Here's how the part is built. I have some questions about the finished solid (model axes, mm). Face numbers are marked on the shaded views. A direction names the side the tool comes from. Round coordinates to 2 decimals unless told otherwise and drop trailing zeros. Loops run counter-clockwise (first coordinate to the right, second up) from the corner with the lowest first, then second, coordinate; pieces in that order, holes last. Notation, with made-up numbers: M 43.5,0.5 L 74.5,0.5 A19 cw 74.5,31.5 Z; hole C 16,66.5 d7. An arc over 180 degrees is marked long. Write each question's results on one line, items separated by ' | '. Start each with the question number.
Autodesk Inventor part; units mm, degrees
ref_plane "YZ Plane" through (0, 0, 0) normal (1, 0, 0) x (0, 1, 0)
ref_plane "XZ Plane" through (0, 0, 0) normal (0, 1, 0) x (-1, 0, 0)
ref_plane "XY Plane" through (0, 0, 0) normal (0, 0, 1) x (1, 0, 0)
sketch "草图1" plane through (0, 0, 0) normal (0, 1, 0) x (-1, 0, 0)
  line L0 (65, 82) -> (-65, 82)
  line L1 (-65, 82) -> (-65, -82)
  line L2 (-65, -82) -> (65, -82)
  line L3 (65, -82) -> (65, 82)
  line L4 (65, 82) -> (-65, -82) construction
  line L5 (-65, 82) -> (65, -82) construction
  point P0 (0, 0)
  dimension "d0" = 130
  dimension "d1" = 164
extrude "拉伸1" add sketch "草图1" along normal blind 15
sketch "草图2" plane through (0, 15, 0) normal (0, 1, 0) x (1, 0, 0)
  line L0 (-40, -82) -> (40, -82)
  line L1 (40, -82) -> (40, 82)
  line L2 (40, 82) -> (-40, 82)
  line L3 (-40, 82) -> (-40, -82)
  line L4 (-40, -82) -> (40, 82) construction
  line L5 (40, -82) -> (-40, 82) construction
  point P0 (0, 0)
  dimension "d4" = 80
  dimension "d5" = 164
extrude "拉伸2" add sketch "草图2" along normal blind 65
sketch "草图3" plane through (0, 0, 0) normal (0, -1, 0) x (1, 0, 0)
  line L0 (34.5, 82) -> (-34.5, 82)
  line L1 (-34.5, 82) -> (-34.5, -82)
  line L2 (-34.5, -82) -> (34.5, -82)
  line L3 (34.5, -82) -> (34.5, 82)
  line L4 (34.5, 82) -> (-34.5, -82) construction
  line L5 (-34.5, 82) -> (34.5, -82) construction
  point P0 (0, 0)
  dimension "d8" = 69
  dimension "d9" = 164
extrude "拉伸3" cut sketch "草图3" against normal blind 20
sketch "草图10" plane through (0, 80, 0) normal (0, 1, 0) x (1, 0, 0)
  line L0 (40, -82) -> (40, 82)
  line L1 (40, 82) -> (-40, 82)
  line L2 (-40, 82) -> (-40, -82)
  line L3 (-40, -82) -> (40, -82)
  arc A0 (10, 6) -> (-10, 6) centre (0, 6) ccw
  circle A1 centre (0, 6) radius 15
  line L4 (40, 82) -> (-40, 82)
  line L5 (-20, 82) -> (-20, -82)
  line L6 (-34.5, -82) -> (34.5, -82)
  line L7 (20, 82) -> (20, -82)
  line L8 (-40, -82) -> (40, -82)
  point P0 (0, 0)
  dimension "d66" = 30
  dimension "d67" = 20
  dimension "d68" = 20
extrude "拉伸4" cut sketch "草图10" against normal blind 4 contours L7 L3 L5 L1
sketch "草图28" plane through (0, 80, -6) normal (0, 1, 0) x (1, 0, 0)
  circle A0 centre (0, 0) radius 15
  point P0 (0, -6)
hole "孔19" at (0, 80, -6) direction (0, -1, 0) diameter 20 depth 25
sketch "草图39" plane through (0, 80, 0) normal (0, 1, 0) x (1, 0, 0)
  line L0 (0, -4) -> (0, 16)
  line L1 (40, 82) -> (20, 82)
  circle A0 centre (30, 45) radius 2.5
  circle A1 centre (30, -20) radius 2.5
  point P0 (0, 0)
  dimension "d287" = 5
  dimension "d289" = 5
  dimension "d290" = 65
extrude "拉伸9" cut sketch "草图39" against normal blind 20
sketch "草图40" plane through (0, 80, 0) normal (0, 1, 0) x (1, 0, 0)
  circle A0 centre (30, 45) radius 2.5
  circle A1 centre (30, 72) radius 4
  point P0 (0, 0)
  dimension "d295" = 8
  dimension "d296" = 27
hole "孔26" at (30, 80, -72) direction (0, -1, 0) diameter 6.647 depth 25
sketch "草图41" plane through (0, 80, 0) normal (0, 1, 0) x (1, 0, 0)
  circle A0 centre (30, -20) radius 2.5
  point P0 (0, 0)
  point P1 (30, -32)
  dimension "d304" = 12
hole "孔27" at (30, 80, 32) direction (0, -1, 0) diameter 6.647 depth 25
mirror "镜像10" about plane through (0, 0, 0) normal (1, 0, 0) of "孔26", "拉伸9", "孔27"
fillet "圆角3" radius 12 4 edges at (-65, 7.5, -82) (-65, 7.5, 82) (65, 7.5, 82) (65, 7.5, -82)
fillet "圆角4" radius 5 8 edges at (20, 78, 82) (20, 78, -82) (40, 47.5, -82) (40, 47.5, 82) (-40, 47.5, 82) (-40, 47.5, -82) (-20, 78, 82) (-20, 78, -82)
sketch "草图42" plane through (-34.5, 20, 82) normal (0, 0, 1) x (1, 0, 0)
  line L0 (69, -20) -> (87.5, -20)
  point P0 (34.5, -20)
  point P1 (34.5, 25)
  dimension "d314" = 45
hole "孔28" at (0, 45, 82) direction (0, 0, -1) diameter 26.211 depth 29 counterbore diameter 32 counterbore depth 10
sketch "草图43" plane through (0, 45, 53) normal (0, 0, 1) x (1, 0, 0)
  circle A0 centre (0, 0) radius 13.1055
  point P0 (0, -45)
hole "孔29" at (0, 45, 53) direction (0, 0, -1) diameter 20 depth 95 counterbore diameter 32 counterbore depth 7
sketch "草图44" plane through (0, 45, -42) normal (0, 0, 1) x (1, 0, 0)
  circle A0 centre (0, 0) radius 10
  point P0 (0, -45)
hole "孔30" at (0, 45, -42) at (0, 45, -42) direction (0, 0, -1) diameter 20.752 end through all counterbore diameter 26 counterbore depth 7
sketch "草图45" plane through (0, 15, 0) normal (0, 1, 0) x (1, 0, 0)
  circle A0 centre (-53, 0) radius 9
  line L0 (0, 16) -> (0, -4)
  circle A1 centre (-53, -70) radius 9
  line L1 (-44, 0) -> (-62, 0)
  circle A2 centre (-53, 70) radius 9
  point P0 (0, 0)
  dimension "d336" = 18
  dimension "d337" = 53
  dimension "d338" = 18
  dimension "d339" = 70
extrude "拉伸10" cut sketch "草图45" against normal blind 2
sketch "草图46" plane through (-53, 13, 70) normal (0, 1, 0) x (1, 0, 0)
  circle A0 centre (0, 0) radius 9
  point P0 (53, 70)
hole "孔31" at (-53, 13, 70) direction (0, -1, 0) diameter 9 end through all
sketch "草图47" plane through (-53, 13, 0) normal (0, 1, 0) x (1, 0, 0)
  circle A0 centre (0, 0) radius 9
  point P0 (53, 0)
hole "孔32" at (-53, 13, 0) direction (0, -1, 0) diameter 9 end through all
sketch "草图48" plane through (-53, 13, -70) normal (0, 1, 0) x (1, 0, 0)
  circle A0 centre (0, 0) radius 9
  point P0 (53, -70)
hole "孔33" at (-53, 13, -70) direction (0, -1, 0) diameter 9 end through all
mirror "镜像11" about plane through (0, 0, 0) normal (1, 0, 0) of "拉伸10", "孔31", "孔32", "孔33"
properties part number "1-夹具体" material "灰口铁"
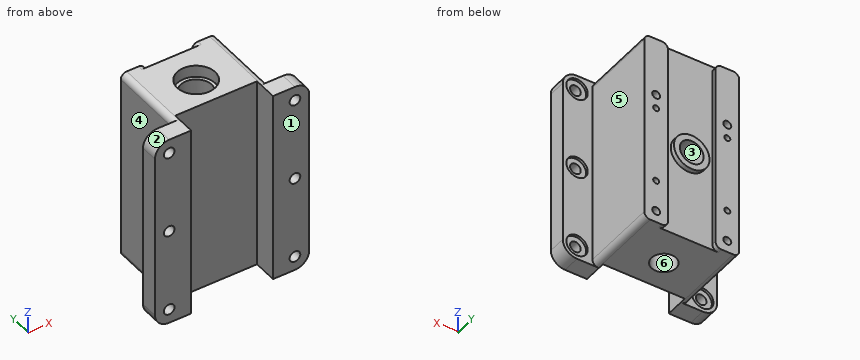
1. I want a section at C-C on y = 68. Count the separate pieces of the cut face and the enclosed holes in it, plus the area to 3 significant figures.
2. I want a section at A-A on z = 32. List the corners of the cut face in (x, y) for me.
3. Which directions (+Z, -Z, +X, -X, +Y, -Y) give clear straight access to the entire face, cutting with the end or side of a thin tool? Please do the marked faces 4, 5 and 6.
4. I need wall thicknesses on line 1 along Z through (x, y) = (53, 13.7); line 2 along X through (y, z) = (4.5, 0); line 3 along Z through (x, y) = (53, 10). Which ranges of each line are inside material? Lowest first, please.
5. I want a section at B-B on x = -30. List the corners of the cut face in (y, z) for me.
6. If we mould it in two halves opening along Z, with no side actions, what happens to the marked faces 1, 2 and 3? For each: released by +Z, released by -Z, zero draft, split by the parting line, or undercut.
7. For pin 1 (3 mm diameter, centred on x = 3, z = -27.5, fed in from +Y); pin 2 (4.5 mm diameter, centred on x = -30, z = -45, fed in from -Y); pin 3 (14.5 mm diameter, centred on x = -53, z = 0, fed in from +Y), each with a flat end and sliding along its axis, tell me the tip position at first contact or that it passes through.
Outcome:
1) separate pieces: 1 | enclosed holes: 9 | area: 12,600 mm2
2) outline: M -65,0 L -34.5,0 L -34.5,20 L 34.5,20 L 34.5,0 L 65,0 L 65,15 L 40,15 L 40,80 L 33.32,80 L 33.32,55 L 26.68,55 L 26.68,80 L 20,80 L 20,76 L -20,76 L -20,80 L -26.68,80 L -26.68,55 L -33.32,55 L -33.32,80 L -40,80 L -40,15 L -65,15 Z; hole C 0,45 d20
3) face 4: +Z, -Z, -X, +Y | face 5: +Z, -Z, +X, +Y | face 6: -Z
4) line 1: -82 to -79, -61 to -9, 9 to 61, 79 to 82 | line 2: -65 to -57.5, -48.5 to -34.5, 34.5 to 48.5, 57.5 to 65 | line 3: -82 to -74.5, -65.5 to -4.5, 4.5 to 65.5, 74.5 to 82
5) outline: M 20,-82 L 80,-82 L 80,-75.32 L 55,-75.32 L 55,-68.68 L 80,-68.68 L 80,-47.5 L 60,-47.5 L 60,-42.5 L 80,-42.5 L 80,17.5 L 60,17.5 L 60,22.5 L 80,22.5 L 80,28.68 L 55,28.68 L 55,35.32 L 80,35.32 L 80,82 L 20,82 Z
6) face 1: zero draft | face 2: released by +Z | face 3: undercut
7) pin 1: y = 76 | pin 2: y = 20 | pin 3: y = 13
